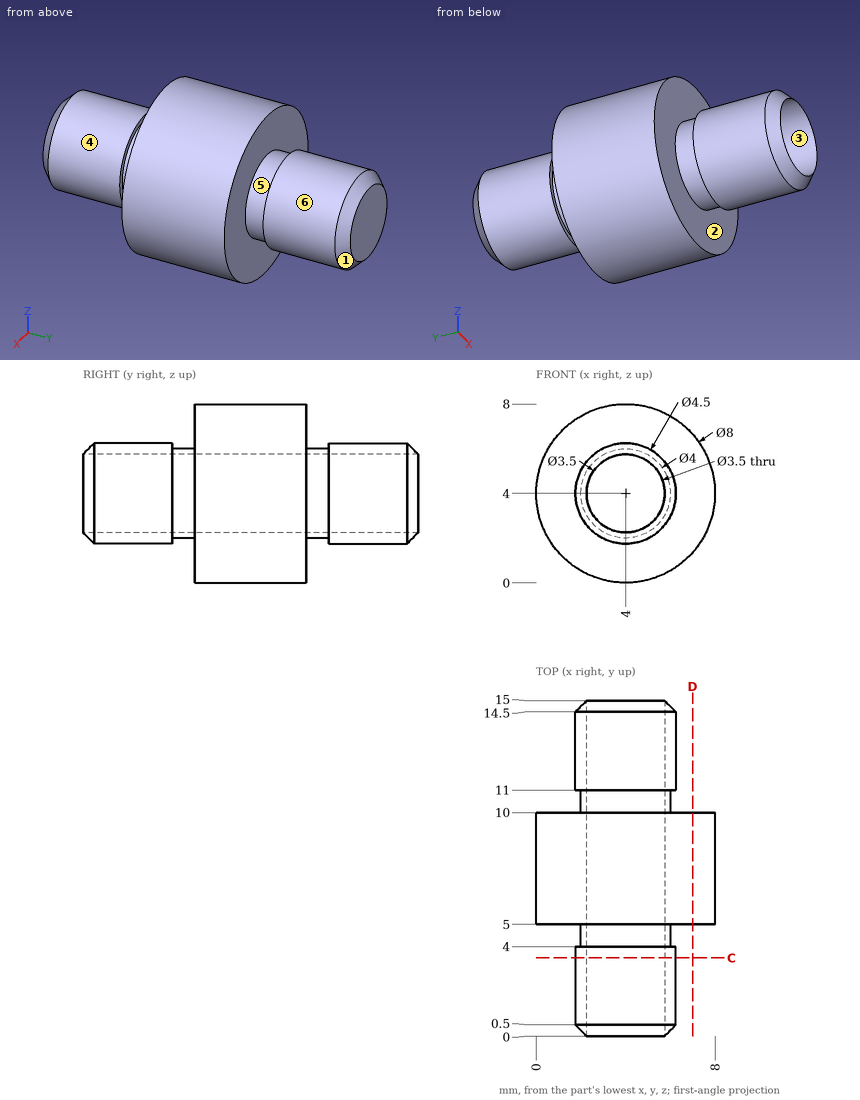
Source: three-view drawing plus pictorial views. Frame: mm from the lowest corner of the part. A direction names the side the tool comes from. Give positions to 0.01 mm unless a question says otherwise; leave off trailing zeros. Order: outer loops, then holes, each group sorted by start corner. A loop starts at its lowest first (then second) coordinate and runs counter-clockwise, first axis right, second up. Notation, with made-up numbers: (-4.5, 64) - (25.5, 64) arc R32 ccw to (25.5, 98) - close; hole circle Ø3 at (55, -36). An arc over 180 degrees is marked (long way). Answer as a JSON object with one key per item and string values. Group by question number.
Q1. Mould query, pull axis X, two halves, no side actions, for the marked faces 1, 2 and 3. Classes: pulls with the +X half, pulls with the -X half, needs draft (parallel to the pull), parting line crosses it, or undercut.
Q2. Cut plane C-C, the plane y = 3.5. Output: boundary loops of the cut face in (x, z).
Q3. Set-up query: the marked faces 4, 5 and 6. Return all of +Z, -Z, +X, -X, +Y, -Y with unobstructed straight access to the full face (end or side cutting, diameter ignored); none if empty.
Q4. First-contact query: pin 1 Ø1.5 at (x, y) = (2.5, 11) entering from -Z; pin 2 Ø2 at (x, z) = (4, 5) entering from -Y; pin 3 Ø1.5 at (x, y) = (5, 12.5) entering from -Z. Flat tips, straight axial feed; report the tip coordinate or a pass-through.
Q5. Line query: probe 1 along Z at (x, y) = (4, 4.75); probe 2 along Z at (x, y) = (4, 8); probe 3 along Y at (x, z) = (6.75, 5). Output: solid intervals per line, ascending.
Q6. Cut plane D-D, the plane x = 7. Output: boundary loops of the cut face in (y, z).
Results:
{
 "1": {"face 1": "parting line crosses it", "face 2": "needs draft", "face 3": "undercut"},
 "2": {"outline": "circle Ø4.5 at (4, 4); hole circle Ø3.5 at (4, 4)"},
 "3": {"face 4": "-Y", "face 5": "none", "face 6": "+Y"},
 "4": {"pin 1": "z = 1.88", "pin 2": "y = 0", "pin 3": "z = 1.76"},
 "5": {"probe 1": "2 to 2.25, 5.75 to 6", "probe 2": "0 to 2.25, 5.75 to 8", "probe 3": "5 to 10"},
 "6": {"outline": "(5, 1.35) - (10, 1.35) - (10, 6.65) - (5, 6.65) - close"}
}
